For this review, take the finished solid that the model builds, in its own axes (mm). A direction names the side the tool comes from. Round coordinates to 2 decimals unless told otherwise and drop trailing zeros. Write each loop counter-clockwise with the first axis right and the second up, starting at its lowest first coordinate (ties: lowest second). Pieces come first, ordered by that corner, then holes. Notation, with made-up numbers: (74, 52) - (125, 52) arc R15 cw to (125, 74) - close; hole circle Ø7 at (81, -34). An arc over 180 degrees is marked (long way). One line per item, written item: value. Start each with the question number.
Q1. For probe 1 along Z at (x, y) = (-26.5, -6.5) (3 decimals); probe 2 along X at (y, z) = (-5, -9); probe 3 along Y at (x, z) = (-29, 12), list the stretches that pass through material, from the lowest coordinate up.
Q2. Add section D-D on x = 11. Write out the cut boundary in (y, z) (3 decimals).
Q3. Add section C-C on x = -13.5. Write out the cut boundary in (y, z) (3 decimals), and give its area (3 significant figures).
Q4. Clearance check with flat-ended pins moving along their axes: pin 1 Ø4 at (y, z) = (-7, -7.5) entering from +X; pin 2 Ø5.5 at (x, y) = (15.5, -7) entering from -Z (3 decimals); pin 3 Ø2 at (x, z) = (-3.5, -7.5) entering from -Y; pin 4 Ø1.5 at (x, y) = (-11, -6.5) entering from -Z. State where each tip first meets the part, or that it passes through.
Q5. Add section B-B on y = -4.75. Write out the cut boundary in (x, z) (3 decimals), and give its area (3 significant figures).
Q6. Tool access review of faces 4 (the face through (6.35, -6, -9)), 5 (the face through (8, -3.81, 8)), 6 (the face through (-12.051, -6, -6)): name each direction out of +Z, -Z, +X, -X, +Y, -Y from which nothing blocks a thin tool from reaching the whole face with its end or side.
Q7. Add section A-A on z = 13.5. Write out the cut boundary in (x, y).
Q8. Mouldability with a two-part tool opening along Z and no side actions: class faces 1 (the face through (0, -2, 3.175)), 2 (the face through (-27.94, -6, 20)), 3 (the face through (-10.6, -6.44, -14.35)) as +Z half, -Z half, draft (parallel to the pull), parting line (faces both ways), or undercut.
```python
from build123d import *

# Parameters (mm, degrees)
F0_W     = 12.7
F0_H     = 6.35
F1_DEPTH = 12.7
F2_R     = 5.08
F3_W     = 24.7787790167
F3_H     = 5.08
F3_W_2   = 24.3673952091
F3_W_3   = 14.3538257742
F4_DEPTH = 31.75
F5_W     = 55.88
F5_H     = 22.86
F6_DEPTH = 25.4


with BuildPart() as f1:
    # F0 (on Front) → F1 (new body)
    with BuildSketch(Plane.XZ):
        Polygon((-6.35, -3.175), (-6.35, 3.175), (-12.0512209833, 3.175), (-12.0512209833, -15.875), (-6.35, -15.875), align=None)
        Rectangle(F0_W, F0_H)
        Polygon((12.4626047909, 3.175), (6.35, 3.175), (6.35, -3.175), (6.35, -15.875), (12.4626047909, -15.875), align=None)
    extrude(amount=F1_DEPTH)

    # F2
    f2_edges = [f1.edges().sort_by_distance(p)[0] for p in [
        (-12.051221, -6.35, 3.175),
        (12.462605, -6.35, 3.175),
        (-12.051221, -6.35, -15.875),
        (12.462605, -6.35, -15.875),
    ]]
    fillet(f2_edges, radius=F2_R)

    # F3 (on face) → F4 (join)
    with BuildSketch(Plane.XY.offset(3.175)):
        with Locations((-19.3606104916, -6.35)):
            Rectangle(F3_W, F3_H)
        with Locations((19.5663023955, -6.35)):
            Rectangle(F3_W_2, F3_H)
        with Locations((0.2056919038, -6.35)):
            Rectangle(F3_W_3, F3_H)
    extrude(amount=F4_DEPTH)

    # F5 (on face) → F6 (cut)
    with BuildSketch(Plane.XZ.offset(8.89)):
        with Locations((0, 19.685)):
            Rectangle(F5_W, F5_H)
    extrude(amount=-F6_DEPTH, mode=Mode.SUBTRACT)


solid = f1.part
```
Result set:
1. probe 1: z = 3.175 to 8.255, 31.115 to 34.925
1. probe 2: x = -12.05 to -6.35, 6.35 to 12.46
1. probe 3: y = -8.89 to -3.81
2. outline: (-12.7, -14.362) - (0, -14.362) - (0, 1.662) - (-12.7, 1.662) - close; (-8.89, 3.175) - (-3.81, 3.175) - (-3.81, 8.255) - (-8.89, 8.255) - close; (-8.89, 31.115) - (-3.81, 31.115) - (-3.81, 34.925) - (-8.89, 34.925) - close
3. outline: (-8.89, 3.175) - (-3.81, 3.175) - (-3.81, 8.255) - (-8.89, 8.255) - close; (-8.89, 31.115) - (-3.81, 31.115) - (-3.81, 34.925) - (-8.89, 34.925) - close
3. area: 45.2 mm^2
4. pin 1: stops at x = 12.46
4. pin 2: stops at z = 3.175
4. pin 3: passes through
4. pin 4: stops at z = -14.68
5. outline: (-31.75, 3.175) - (-6.971, 3.175) arc R5.08 ccw to (-12.051, -1.905) - (-12.051, -10.795) arc R5.08 ccw to (-6.971, -15.875) - (-6.35, -15.875) - (-6.35, -3.175) - (6.35, -3.175) - (6.35, -15.875) - (7.383, -15.875) arc R5.08 ccw to (12.463, -10.795) - (12.463, -1.905) arc R5.08 ccw to (7.383, 3.175) - (31.75, 3.175) - (31.75, 34.925) - (-31.75, 34.925) - close; hole (-27.94, 8.255) - (27.94, 8.255) - (27.94, 31.115) - (-27.94, 31.115) - close
5. area: 1,020 mm^2
6. face 4: -Z, +Y, -Y
6. face 5: +Z, +X, -X, +Y
6. face 6: -Z, -X, +Y, -Y
7. outline: (-31.75, -8.89) - (-27.94, -8.89) - (-27.94, -3.81) - (-31.75, -3.81) - close; (27.94, -8.89) - (31.75, -8.89) - (31.75, -3.81) - (27.94, -3.81) - close
8. face 1: +Z half
8. face 2: undercut
8. face 3: -Z half
